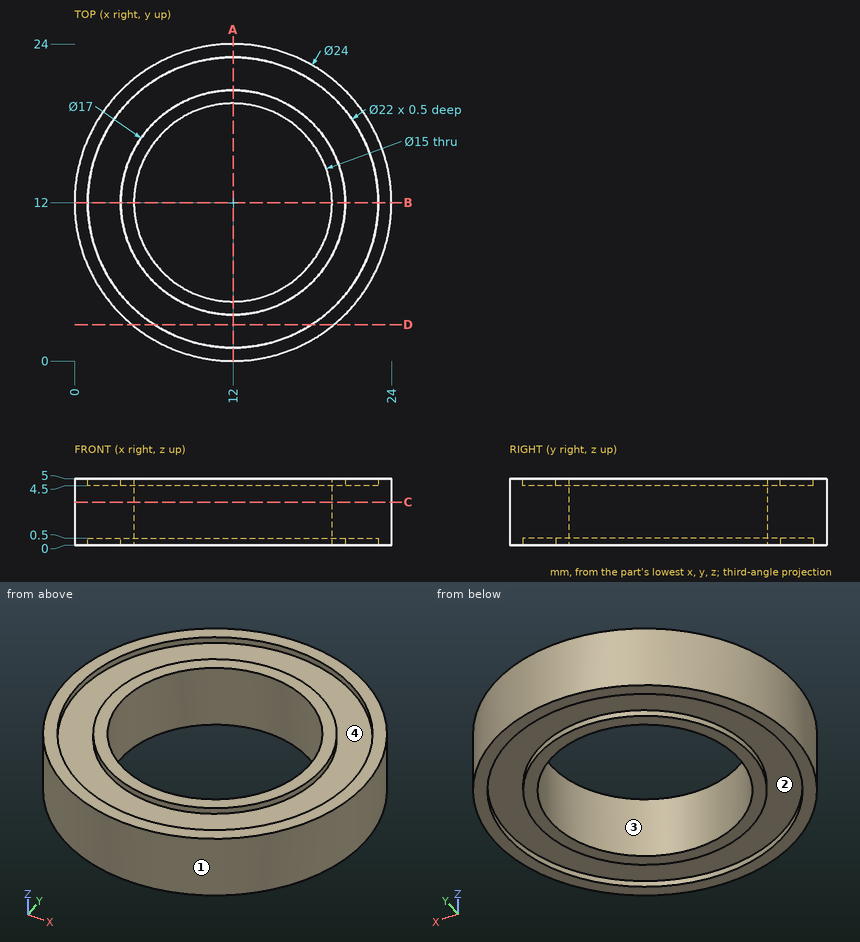
Design review of the part shown in the three views and the two pictorial views. Dimensions are in mm from the part's minimum x, y and z. A direction names the side the tool comes from. Coordinates: 2 decimals unless noted, no trailing zeros. Loops run counter-clockwise (first coordinate to the right, second up) from the corner with the lowest first, then second, coordinate; pieces in that order, holes last.
(1) Insertion check: P1, Ø9, axis at x = 12, y = 12, coming from the +Z side; P2, Ø1.5, axis at x = 7, y = 3.5, coming from the -Z side; P3, Ø2, axis at x = 17.5, z = 0.5, coming from the +Y side; P4, Ø3, axis at x = 17.5, y = 15, coming from the -Z side. Each pin has a flat end and moves straight along its axis. Give the tip position at first contact, or say it passes through.
Determined:
P1: passes through
P2: stops at z = 0.5
P3: stops at y = 23.12
P4: stops at z = 0
(2) Draft analysis for pull direction Y (two halves, no side actions). For the marked faces 1 and 2, state which applies: +Y half, -Y half, draft (parallel to the pull), parting line (faces both ways), or undercut.
Determined:
face 1: parting line
face 2: undercut
(3) Consider section C-C, the plane z = 3.25. Give the boundary of the cut face in (x, y).
Determined:
outline: circle Ø24 at (12, 12); hole circle Ø15 at (12, 12)
(4) Tool access review of the marked faces 3 and 4: name each direction out of +Z, -Z, +X, -X, +Y, -Y from which nothing blocks a thin tool from reaching the whole face with its end or side.
Determined:
face 3: +Z, -Z
face 4: +Z
(5) Consider section A-A, the plane x = 12. Give the boundary of the cut face in (y, z).
Determined:
outline: (0, 0) - (1, 0) - (1, 0.5) - (3.5, 0.5) - (3.5, 0) - (4.5, 0) - (4.5, 5) - (3.5, 5) - (3.5, 4.5) - (1, 4.5) - (1, 5) - (0, 5) - close; (19.5, 0) - (20.5, 0) - (20.5, 0.5) - (23, 0.5) - (23, 0) - (24, 0) - (24, 5) - (23, 5) - (23, 4.5) - (20.5, 4.5) - (20.5, 5) - (19.5, 5) - close
(6) Consider section D-D, the plane y = 2.75. Give the boundary of the cut face in (x, z).
Determined:
outline: (4.36, 0) - (6.05, 0) - (6.05, 0.5) - (17.95, 0.5) - (17.95, 0) - (19.64, 0) - (19.64, 5) - (17.95, 5) - (17.95, 4.5) - (6.05, 4.5) - (6.05, 5) - (4.36, 5) - close
(7) Wall thickness on L1, parallel to Y at x = 12, z = 4.85; L2, parallel to X at y = 12.25, z = 3.35; L3, parallel to Z at x = 20.5, y = 11.25: over which ranges is each line inside the solid? List them lowest first.
Determined:
L1: y = 0 to 1, 3.5 to 4.5, 19.5 to 20.5, 23 to 24
L2: x = 0 to 4.5, 19.5 to 24
L3: z = 0.5 to 4.5
